Input: part model. Units: mm. Frame: model coordinates. Face numbers are marked on the shaded views. A direction names the side the tool comes from. Coordinates: 2 decimals unless noted, no trailing zeros. Order: outer loops, then holes, each group sorted by start corner. A loop starts at its lowest first (then second) coordinate and runs counter-clockwise, first axis right, second up. Notation, with made-up numbers: M -25.5,69 L -10.5,69 A30 ccw -10.5,102 Z; hole C 78,24 d1. An arc over 180 degrees is marked long. One line per item, written item: value.
```python
from build123d import *

# Parameters (mm, degrees)
F0_W        = 101.2
F0_H        = 101.2
F1_DEPTH    = 100
F2_T        = -1.2
F4_W        = 0.8
F4_H        = 0.8
F5_DEPTH    = 100.001
F6_R        = 1.2
F7_T4_DEPTH = 101.8
F8_R        = 2.4
F9_T1_DEPTH = 110.8
F12_DEPTH   = 25
F14_DEPTH   = 25


# Not quite as in the source:
# - a fillet or chamfer that OpenCascade refuses, or shapes differently, is made with other operations: its cross-section is extruded or revolved along the edge and cut away or added


with BuildPart() as f1:
    # F0 (on Top) → F1 (new body)
    with BuildSketch(Plane.XY):
        Rectangle(F0_W, F0_H)
    extrude(amount=F1_DEPTH)

    # F2
    f2_openings = [f1.faces().sort_by_distance(p)[0] for p in [
        (0, 0, 100),
        (0, -50.6, 50),
        (50.6, 0, 50),
    ]]
    offset(amount=F2_T, openings=f2_openings)

    # F4 (on face) → F5 (cut, through all)
    with BuildSketch(Plane.XY.offset(100)):
        with Locations((-49, 49)):
            Rectangle(F4_W, F4_H)
        Polygon((-50.6, 50.6), (-50.6, 48.6), (-49.4, 48.6), (-49.4, 49.4), (-48.6, 49.4), (-48.6, 50.6), align=None)
    extrude(amount=-F5_DEPTH, mode=Mode.SUBTRACT)

    # F6
    f6_edges = [f1.edges().sort_by_distance(p)[0] for p in [
        (1, 49.4, 1.2),
    ]]
    fillet(f6_edges, radius=F6_R)

    # F7: fillet of radius 1.2 on 1 edges, made by hand


with BuildPart() as f7_tool2:
    # F7_s3 → F7_t4 (new body)
    with BuildSketch(Plane.XZ.offset(50.6)):
        with BuildLine():
            ThreePointArc((-49.4, 2.4), (-49.0485281374, 1.5514718626), (-48.2, 1.2))
            Line((-48.2, 1.2), (-49.4, 1.2))
            Line((-49.4, 1.2), (-49.4, 2.4))
        make_face()
    extrude(amount=-F7_T4_DEPTH)

    split(bisect_by=Plane.XZ.offset(-48.6), keep=Keep.TOP)


with BuildPart() as f1_1:
    add(f1.part)

    # F7_t1: union F7_tool2
    add(f7_tool2.part)

    # F8
    f8_edges = [f1_1.edges().sort_by_distance(p)[0] for p in [
        (-50.6, -1, 0),
    ]]
    fillet(f8_edges, radius=F8_R)

    # F9: fillet of radius 2.4 on 1 edges, made by hand

    # F9_s2 → F9_t1 (cut)
    with BuildSketch(Plane.YZ.offset(-54.2)):
        with BuildLine():
            ThreePointArc((50.6, 2.4), (49.8970562748, 0.7029437252), (48.2, 0))
            Line((48.2, 0), (50.6, 0))
            Line((50.6, 0), (50.6, 2.4))
        make_face()
    extrude(amount=F9_T1_DEPTH, mode=Mode.SUBTRACT)

    # F11 (on face) → F12 (cut)
    with BuildSketch(Plane(origin=(0, 50.6, 0), x_dir=(-1, 0, 0), z_dir=(0, 1, 0))):
        Polygon((-11.4, 100), (-50.6, 100), (-50.6, 30), align=None)
    extrude(amount=-F12_DEPTH, mode=Mode.SUBTRACT)

    # F13 (on face) → F14 (cut)
    with BuildSketch(Plane(origin=(0, 0, 0), x_dir=(1, 0, 0), z_dir=(0, 0, -1))):
        Polygon((50.6, -48.2), (50.6, 50.6), (-48.2, 50.6), align=None)
    extrude(amount=-F14_DEPTH, mode=Mode.SUBTRACT)


solid = f1_1.part
```
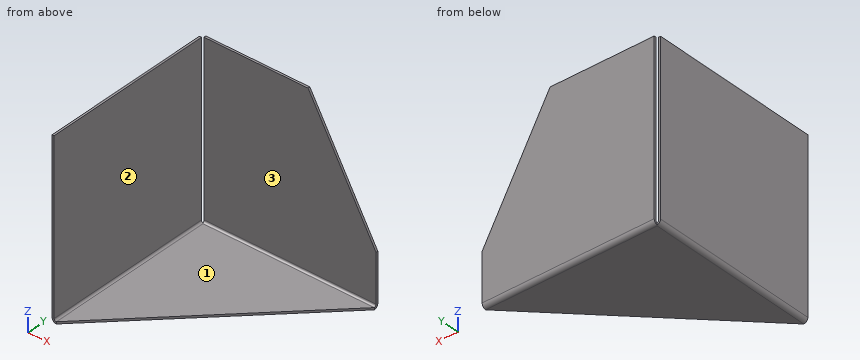
(1) Cut plane A-A on z = 23.5. Output: boundary loops of the cut face in (x, y).
Data:
outline: M -50.6,-50.6 L -49.4,-50.6 L -49.4,48.6 L -50.6,48.6 Z; M -48.6,49.4 L 50.6,49.4 L 50.6,50.6 L -48.6,50.6 Z
(2) Ray query, line 1 (X direction, y = 27.5, z = 46.5); line 2 (Y direction, x = -12, z = 44); line 3 (Z direction, x = -28.5, y = -14). Return the intervals inside material, ascending. Write a range as from..to.
Data:
line 1: x = -50.6..-49.4
line 2: y = 49.4..50.6
line 3: z = 0..1.2
(3) Access query for the marked faces 1, 2 and 3. Directions: +Z, -Z, +X, -X, +Y, -Y. A direction counts if a zero-diameter tool reaches every point of the face in a straight line with its end or side. Return the directions, or none.
Data:
face 1: +Z, +X, -Y
face 2: +Z, +X, +Y, -Y
face 3: +Z, +X, -X, -Y
(4) First-contact query: pin 1 (3 mm diameter, centred on x = -16.5, z = 56.5, fed in from -Y); pin 2 (5 mm diameter, centred on x = -19.5, y = -21, fed in from +Z); pin 3 (1 mm diameter, centred on y = -27.5, z = 67, fed in from +X); pin 4 (10 mm diameter, centred on x = 3, y = -8, fed in from -Z). Flat tips, straight axial feed; report the tip coordinate or a pass-through.
Data:
pin 1: stops at y = 49.4
pin 2: stops at z = 1.2
pin 3: stops at x = -49.4
pin 4: passes through
(5) Cut plane B-B on x = -37.5. Output: boundary loops of the cut face in (y, z).
Data:
outline: M -39.9,0 L 48.2,0 A2.4 ccw 50.6,2.4 L 50.6,100 L 49.4,100 L 49.4,2.4 A1.2 cw 48.2,1.2 L -39.9,1.2 Z
(6) Cut plane D-D on z = 56. Output: boundary loops of the cut face in (x, y), plus the area to 3 significant figures.
Data:
outline: M -50.6,-50.6 L -49.4,-50.6 L -49.4,48.6 L -50.6,48.6 Z; M -48.6,49.4 L 36.04,49.4 L 36.04,50.6 L -48.6,50.6 Z
area: 221 mm2
(7) Cut plane C-C on y = -10. Output: boundary loops of the cut face in (x, z), plus the area to 3 significant figures.
Data:
outline: M -50.6,2.4 A2.4 ccw -48.2,0 L -7.6,0 L -7.6,1.2 L -48.2,1.2 A1.2 cw -49.4,2.4 L -49.4,100 L -50.6,100 Z
area: 169 mm2
